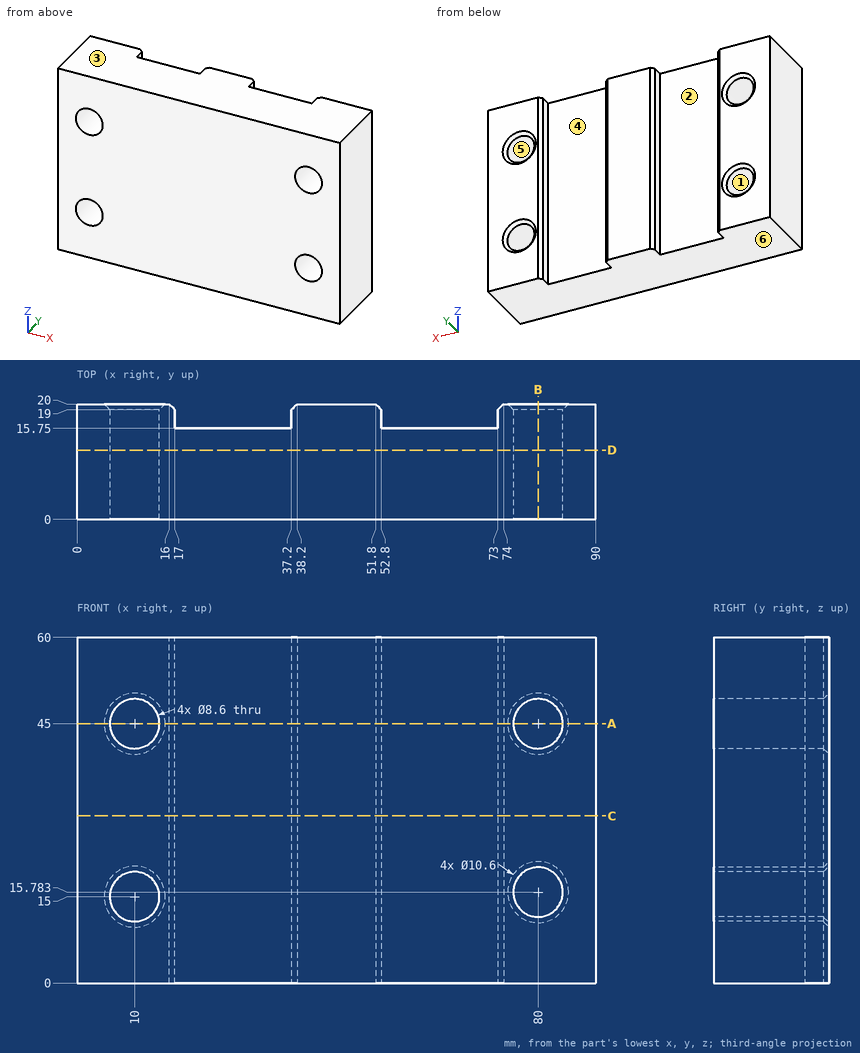
Input: dimensioned drawing with shaded views. Units: mm. Origin: part minimum x, y, z. A direction names the side the tool comes from. Coordinates: 2 decimals unless noted, no trailing zeros. Loops run counter-clockwise (first coordinate to the right, second up) from the corner with the lowest first, then second, coordinate; pieces in that order, holes last. Notation, with made-up numbers: M 9,17.5 L 45,17.5 A23 ccw 45,36.5 Z; hole C -30,68 d7. An arc over 180 degrees is marked long. Use a Markdown table: item, result. Add a question column.
Q1. Access query for the marked faces 1 and 2. Directions: +Z, -Z, +X, -X, +Y, -Y. A direction counts if a zero-diameter tool reaches every point of the face in a straight line with its end or side. Return the directions, or none.
Q2. Section query B-B, the plane x = 80. Return loops of the section in (y, z).
Q3. First-contact query: pin 1 (6 mm diameter, centred on x = 25.5, z = 33, fed in from +Y). Flat tip, straight axial feed; report the tip coordinate or a pass-through.
Q4. Draft query along Z for the marked faces 3, 4, 5 and 6. Return one class per face: pulls with the +Z half, pulls with the -Z half, needs draft (parallel to the pull), parting line crosses it, or undercut.
Q5. Material intervals for L1, parallel to Z at x = 80, y = 8.5; L2, parallel to Z at x = 10, y = 10.25; L3, parallel to X at y = 16.5, z = 30, sorted ascending.
Q6. Section query A-A, the plane z = 45. Return loops of the section in (x, y).
Q7. Section query D-D, the plane y = 12. Return loops of the section in (x, z).
Q8. Section query C-C, the plane z = 29. Return loops of the section in (x, y).
Result:
| question | item | result |
|---|---|---|
| 1 | face 1 | +Y, -Y |
| 1 | face 2 | +Z, -Z, +Y |
| 2 | outline | M 0,0 L 20,0 L 20,10.48 L 19,11.48 L 0,11.48 Z; M 0,20.08 L 19,20.08 L 20,21.08 L 20,39.7 L 19,40.7 L 0,40.7 Z; M 0,49.3 L 19,49.3 L 20,50.3 L 20,60 L 0,60 Z |
| 3 | pin 1 | stops at y = 15.75 |
| 4 | face 3 | pulls with the +Z half |
| 4 | face 4 | needs draft |
| 4 | face 5 | undercut |
| 4 | face 6 | pulls with the -Z half |
| 5 | L1 | z = 0 to 11.48, 20.08 to 40.7, 49.3 to 60 |
| 5 | L2 | z = 0 to 10.7, 19.3 to 40.7, 49.3 to 60 |
| 5 | L3 | x = 0 to 17, 37.2 to 52.8, 73 to 90 |
| 6 | outline | M 0,0 L 5.7,0 L 5.7,19 L 4.7,20 L 0,20 Z; M 14.3,0 L 75.7,0 L 75.7,19 L 74.7,20 L 74,20 L 73,19 L 73,15.75 L 52.8,15.75 L 52.8,19 L 51.8,20 L 38.2,20 L 37.2,19 L 37.2,15.75 L 17,15.75 L 17,19 L 16,20 L 15.3,20 L 14.3,19 Z; M 84.3,0 L 90,0 L 90,20 L 85.3,20 L 84.3,19 Z |
| 7 | outline | M 0,0 L 90,0 L 90,60 L 0,60 Z; hole C 10,15 d8.6; hole C 10,45 d8.6; hole C 80,15.78 d8.6; hole C 80,45 d8.6 |
| 8 | outline | M 0,0 L 90,0 L 90,20 L 74,20 L 73,19 L 73,15.75 L 52.8,15.75 L 52.8,19 L 51.8,20 L 38.2,20 L 37.2,19 L 37.2,15.75 L 17,15.75 L 17,19 L 16,20 L 0,20 Z |
